For this review, take the finished solid that the model builds, in its own axes (mm). A direction names the side the tool comes from. Give positions to 0.01 mm unless a question says otherwise; leave off trailing zeros. Loops run counter-clockwise (first coordinate to the right, second up) from the corner with the lowest first, then second, coordinate; pieces in that order, holes last. Notation, with made-up numbers: (-34, -14) -> (3, -14) arc R37 cw to (3, 25) -> close; hole circle Ø4 at (6.5, 35). An arc over 180 degrees is marked (long way). Answer as CSV lines item,"result". Start each with the question number.
Item 1: Clearance check with flat-ended pins moving along their axes: P1, Ø3, axis at y = 2.5, z = 6, coming from the +X side; P2, Ø1, axis at x = -11, y = 2, coming from the -Z side; P3, Ø2.5, axis at x = -6, y = 1.5, coming from the +Z side. State where each tip first meets the part, or that it passes through.
Item 2: Add section D-D on z = -2. State the section outline as (x, y) points.
Item 3: Machinability: for faces 4 (the face through (0, 2, 5)), 5 (the face through (-11, 3.7, -3)), 6 (the face through (-1, 0.65, 3)), which of the approach directions +Z, -Z, +X, -X, +Y, -Y give a long, thin tool a straight path to every point of the face, cutting with its end or side? Answer none if there is none.
Item 4: Add section A-A on z = 4.5. State the section outline as (x, y) points, plus the area to 3 significant figures.
Item 5: The part is to be moulded in two halves that separate along Y. For faces 1 (the face through (10.95, -2, -1)), 2 (the face through (0.55, -1, 3)), 3 (the face through (-11, 4.6, -2)), say which applies: +Y half, -Y half, draft (parallel to the pull), parting line (faces both ways), or undercut.
Item 6: Add section C-C on z = -0.5. State the section outline as (x, y) points, plus the area to 3 significant figures.
Item 7: Add section B-B on x = -12.75. State the section outline as (y, z) points, plus the area to 3 significant figures.
Item 8: For L1, parallel to Y at x = 0, z = 4.2; L2, parallel to X at y = 3, z = -1.25; L3, parallel to X at y = 2.5, z = -1, list the stretches that pass through material, from the lowest coordinate up. Write a range as from..to.
```python
from build123d import *

# Parameters (mm, degrees)
SKETCH1_R               = 3.9
SKETCH1_R_2             = 3
SKETCH1_W               = 1.45
SKETCH1_H               = 1.3
SKETCH1_W_2             = 1.1
SKETCH1_H_2             = 1.35
BOSS_EXTRUDE1_DEPTH     = 7
SKETCH2_R               = 3
BOSS_EXTRUDE2_DEPTH     = 3
SKETCH4_W               = 30
SKETCH4_H               = 7.8
BOSS_EXTRUDE3_DEPTH     = 4.2
SKETCH3_W               = 1.45
SKETCH3_H               = 1.35
CUT_EXTRUDE3_DEPTH      = 18.180221186
CUT_EXTRUDE3_DEPTH_BACK = 18.180221186
SKETCH5_W               = 15.6
SKETCH5_H               = 7.8
CUT_EXTRUDE4_DEPTH      = 3
SKETCH6_W               = 2.25
SKETCH6_H               = 6.7
CUT_EXTRUDE5_DEPTH      = 3
CUT_EXTRUDE6_DEPTH      = 3
SKETCH8_W               = 2.25
SKETCH8_H               = 7.6
CUT_EXTRUDE7_DEPTH      = 0.4
FILLET1_R               = 1
CHAMFER1_SIZE           = 0.3


with BuildPart() as part:
    # Sketch1 → Boss-Extrude1 (new body)
    with BuildSketch(Plane.XY):
        Circle(SKETCH1_R)
        Circle(SKETCH1_R_2, mode=Mode.SUBTRACT)
        with Locations((-1.275, 0)):
            Rectangle(SKETCH1_W, SKETCH1_H)
        with Locations((0, -1.325)):
            Rectangle(SKETCH1_W_2, SKETCH1_H_2)
        Rectangle(SKETCH1_W_2, SKETCH1_H)
        with Locations((1.275, 0)):
            Rectangle(SKETCH1_W, SKETCH1_H)
        with Locations((0, 1.325)):
            Rectangle(SKETCH1_W_2, SKETCH1_H_2)
    extrude(amount=BOSS_EXTRUDE1_DEPTH)

    # Sketch2 → Boss-Extrude2 (add)
    with BuildSketch(Plane.XY):
        Circle(SKETCH2_R)
    extrude(amount=BOSS_EXTRUDE2_DEPTH)

    # Sketch4 → Boss-Extrude3 (add)
    with BuildSketch(Plane.XY):
        Polygon((-15, 4.6), (-15, 3.9), (-7.8, 3.9), (-8.92023417, 4.6), align=None)
        Rectangle(SKETCH4_W, SKETCH4_H)
        Polygon((8.92023417, 4.6), (7.8, 3.9), (15, 3.9), (15, 4.6), align=None)
    extrude(amount=-BOSS_EXTRUDE3_DEPTH)

    # Sketch3 → Cut-Extrude3 (cut, two sides)
    with BuildSketch(Plane.XY) as cut_extrude3_sk:
        with Locations((-1.275, 1.325)):
            Rectangle(SKETCH3_W, SKETCH3_H)
        with Locations((1.275, -1.325)):
            Rectangle(SKETCH3_W, SKETCH3_H)
    extrude(amount=CUT_EXTRUDE3_DEPTH, mode=Mode.SUBTRACT)
    extrude(cut_extrude3_sk.sketch, amount=-CUT_EXTRUDE3_DEPTH_BACK, mode=Mode.SUBTRACT)

    # Sketch5 → Cut-Extrude4 (cut)
    with BuildSketch(Plane(origin=(0, 0, -4.2), x_dir=(-1, 0, 0), z_dir=(0, 0, -1))):
        Rectangle(SKETCH5_W, SKETCH5_H)
    extrude(amount=-CUT_EXTRUDE4_DEPTH, mode=Mode.SUBTRACT)

    # Sketch6 → Cut-Extrude5 (cut)
    with BuildSketch(Plane.XY):
        with Locations((12.975, 0.35)):
            Rectangle(SKETCH6_W, SKETCH6_H)
        with Locations((-12.975, 0.35)):
            Rectangle(SKETCH6_W, SKETCH6_H)
    extrude(amount=-CUT_EXTRUDE5_DEPTH, mode=Mode.SUBTRACT)

    # Sketch7 → Cut-Extrude6 (cut)
    with BuildSketch(Plane(origin=(0, 0, -4.2), x_dir=(-1, 0, 0), z_dir=(0, 0, -1))):
        Polygon((12.06, -3), (10.95, -3), (10.95, -3.9), (8.7, -3.9), (8.7, 3.7), (14.1, 3.7), (14.1, 1.7), (12.06, 1.7), align=None)
        Polygon((-8.7, 3.7), (-14.1, 3.7), (-14.1, 1.7), (-12.06, 1.7), (-12.06, -3), (-10.95, -3), (-10.95, -3.9), (-8.7, -3.9), align=None)
    extrude(amount=-CUT_EXTRUDE6_DEPTH, mode=Mode.SUBTRACT)

    # Sketch8 → Cut-Extrude7 (cut)
    with BuildSketch(Plane(origin=(0, 0, -1.2), x_dir=(-1, 0, 0), z_dir=(0, 0, -1))):
        with Locations((-9.825, -0.1)):
            Rectangle(SKETCH8_W, SKETCH8_H)
        with Locations((9.825, -0.1)):
            Rectangle(SKETCH8_W, SKETCH8_H)
    extrude(amount=-CUT_EXTRUDE7_DEPTH, mode=Mode.SUBTRACT)

    # Fillet1
    fillet1_edges = [part.edges().sort_by_distance(p)[0] for p in [
        (-15, 4.6, -2.1),
        (15, 4.6, -2.1),
        (15, -3.9, -2.1),
        (-15, -3.9, -2.1),
    ]]
    fillet(fillet1_edges, radius=FILLET1_R)

    # Chamfer1
    chamfer1_edges = [part.edges().sort_by_distance(p)[0] for p in [
        (-2, 0, 7),
        (-1.275, -0.65, 7),
        (-0.55, -1.325, 7),
        (0, -2, 7),
        (0.55, -1.325, 7),
        (1.275, -0.65, 7),
        (-0.55, 1.325, 7),
        (2, 0, 7),
        (1.275, 0.65, 7),
        (0.55, 1.325, 7),
        (0, 2, 7),
        (-1.275, 0.65, 7),
    ]]
    chamfer(chamfer1_edges, length=CHAMFER1_SIZE)


solid = part.part
```
Computed values:
1,P1,"x = 3.77"
1,P2,"z = -1.2"
1,P3,"z = 0"
2,outline,"(-15, -2.9) arc R1 ccw to (-14, -3.9) -> (-10.95, -3.9) -> (-10.95, -3) -> (-14.1, -3) -> (-14.1, 3.7) -> (-8.7, 3.7) -> (-8.7, -3.9) -> (-7.8, -3.9) -> (-7.8, 3.9) -> (-8.92, 4.6) -> (-14, 4.6) arc R1 ccw to (-15, 3.6) -> close; (7.8, -3.9) -> (8.7, -3.9) -> (8.7, 3.7) -> (14.1, 3.7) -> (14.1, -3) -> (10.95, -3) -> (10.95, -3.9) -> (14, -3.9) arc R1 ccw to (15, -2.9) -> (15, 3.6) arc R1 ccw to (14, 4.6) -> (8.92, 4.6) -> (7.8, 3.9) -> close"
3,face 4,"+Z"
3,face 5,"-Z"
3,face 6,"+Z, -Z"
4,outline,"circle Ø7.8 at (0, 0); (-2, -0.65) -> (-0.55, -0.65) -> (-0.55, -2) -> (0.55, -2) -> (0.55, -0.65) -> (2, -0.65) -> (2, 0.65) -> (0.55, 0.65) -> (0.55, 2) -> (-0.55, 2) -> (-0.55, 0.65) -> (-2, 0.65) -> close; hole circle Ø6 at (0, 0)"
4,area,"27.7 mm²"
5,face 1,"draft"
5,face 2,"undercut"
5,face 3,"+Y half"
6,outline,"(-15, -2.9) arc R1 ccw to (-14, -3.9) -> (14, -3.9) arc R1 ccw to (15, -2.9) -> (15, 3.6) arc R1 ccw to (14, 4.6) -> (8.92, 4.6) -> (7.8, 3.9) -> (-7.8, 3.9) -> (-8.92, 4.6) -> (-14, 4.6) arc R1 ccw to (-15, 3.6) -> close; hole (-14.1, -3) -> (-11.85, -3) -> (-11.85, 3.7) -> (-14.1, 3.7) -> close; hole (-2, 0.65) -> (-0.55, 0.65) -> (-0.55, 2) -> (-2, 2) -> close; hole (0.55, -2) -> (2, -2) -> (2, -0.65) -> (0.55, -0.65) -> close; hole (11.85, -3) -> (14.1, -3) -> (14.1, 3.7) -> (11.85, 3.7) -> close"
6,area,"208 mm²"
7,outline,"(-3.9, -4.2) -> (1.7, -4.2) -> (1.7, -3) -> (-3, -3) -> (-3, 0) -> (-3.9, 0) -> close; (3.7, -4.2) -> (4.6, -4.2) -> (4.6, 0) -> (3.7, 0) -> close"
7,area,"13.2 mm²"
8,L1,"-3.9..-3, -2..2, 3..3.9"
8,L2,"-15..-14.1, -8.7..-7.8, 7.8..8.7, 14.1..15"
8,L3,"-15..-14.1, -11.85..-10.95, -8.7..8.7, 10.95..11.85, 14.1..15"
